Source: three-view drawing plus pictorial views. Frame: mm from the lowest corner of the part. A direction names the side the tool comes from. Give positions to 0.01 mm unless a question says otherwise; leave off trailing zeros. Order: outer loops, then holes, each group sorted by start corner. A loop starts at its lowest first (then second) coordinate and runs counter-clockwise, first axis right, second up. Notation, with made-up numbers: M -22.75,-15 L 0.25,-15 A24 cw 0.25,3 Z; hole C -14,47.25 d5. An arc over 180 degrees is marked long. Use CSV: the item, a comma, the result in double quotes.
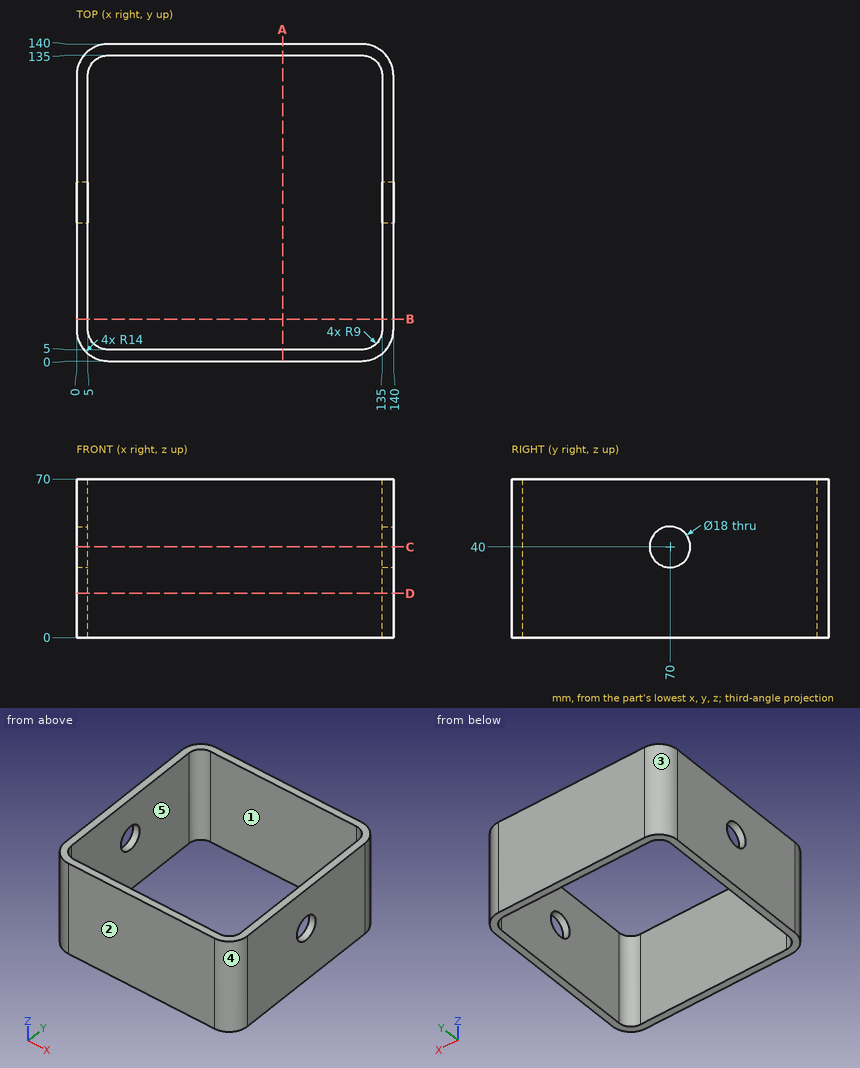
1. Section D-D, the plane z = 19.5. Return the cut outline in (x, y).
Answer:
outline,"M 0,14 A14 ccw 14,0 L 126,0 A14 ccw 140,14 L 140,126 A14 ccw 126,140 L 14,140 A14 ccw 0,126 Z; hole M 5,14 A9 ccw 14,5 L 126,5 A9 ccw 135,14 L 135,126 A9 ccw 126,135 L 14,135 A9 ccw 5,126 Z"
2. Reachability of the marked faces 1 and 2 from +Z, -Z, +X, -X, +Y, -Y: full face, straight path, thin tool, end or side. Return the list, or none.
Answer:
face 1,"+Z, -Z"
face 2,"+Z, -Z, +X, -X, -Y"
3. Line query: line 1 (X direction, y = 91, z = 31.5); line 2 (Z direction, x = 138, y = 70). Output: solid intervals per line, ascending.
Answer:
line 1,"0 to 5, 135 to 140"
line 2,"0 to 31, 49 to 70"
4. Pull-direction query (Y, two-part tool) for the marked faces 3, 4 and 5; classes: +Y half, -Y half, draft (parallel to the pull), parting line (faces both ways), or undercut.
Answer:
face 3,"+Y half"
face 4,"-Y half"
face 5,"undercut"
5. Section C-C, the plane z = 40. Return the cut outline in (x, y).
Answer:
outline,"M 0,14 A14 ccw 14,0 L 126,0 A14 ccw 140,14 L 140,61 L 135,61 L 135,14 A9 cw 126,5 L 14,5 A9 cw 5,14 L 5,61 L 0,61 Z; M 0,79 L 5,79 L 5,126 A9 cw 14,135 L 126,135 A9 cw 135,126 L 135,79 L 140,79 L 140,126 A14 ccw 126,140 L 14,140 A14 ccw 0,126 Z"
6. Pin query (flat end, axial travel): pin 1 Ø21 at (x, z) = (79, 31.5) entering from -Y; pin 2 Ø11 at (y, z) = (70, 40) entering from +X. Return the tip coordinate at first contact, or that it passes through.
Answer:
pin 1,"y = 0"
pin 2,"through"
7. Section A-A, the plane x = 91. Return the cut outline in (y, z), plus the area to 3 significant figures.
Answer:
outline,"M 0,0 L 5,0 L 5,70 L 0,70 Z; M 135,0 L 140,0 L 140,70 L 135,70 Z"
area,"700 mm2"
